Model file for the job. Use its own axes, mm. Coordinates: 2 decimals unless noted, no trailing zeros. Write each loop counter-clockwise with the first axis right and the second up, starting at its lowest first coordinate (ties: lowest second). Pieces come first, ordered by that corner, then holes. Notation, with made-up numbers: M 85.25,21.5 L 127.25,21.5 A3 cw 127.25,25.5 Z; hole C 25.25,17 d9. An arc over 180 degrees is marked long. One line per question, with ' | ' between items. Start each with the question number.
(1) Two-plate mould, pull along X, no slides. Class faces 1 (the face through (3.19, -39.37, 1.97)), 2 (the face through (103, 25, 4)), 3 (the face through (-28.24, 37.62, 1.97)): +X half, -X half, draft (parallel to the pull), parting line (faces both ways), or undercut.
(2) Wall check: probe 1 along Y at (x, z) = (56, 1.4); probe 2 along X at (y, z) = (4, 1.55); probe 3 along X at (y, z) = (-11, 0.2). Give the ranges that are in metal, low to high.
(3) Cut at A-A (z = 1.35). Write the cut outline in (x, y), plus the area to 3 significant figures.
(4) Cut at B-B (x = 131). Write the cut outline in (y, z).
(5) Cut at C-C (y = 32). Write the cut outline in (x, z).
(6) Flat gauge pins, fed straight in: pin 1 Ø1.2 at (y, z) = (4.5, 2) entering from +X; pin 2 Ø2 at (y, z) = (-7, 2.5) entering from -X. Where does each tip first touch, or does it go through?
Autodesk Inventor part; units mm, degrees
ref_plane "YZ Plane" through (0, 0, 0) normal (1, 0, 0) x (0, 1, 0)
ref_plane "XZ Plane" through (0, 0, 0) normal (0, 1, 0) x (-1, 0, 0)
ref_plane "XY Plane" through (0, 0, 0) normal (0, 0, 1) x (1, 0, 0)
sketch "Sketch1" plane through (0, 0, 0) normal (0, 0, 1) x (1, 0, 0)
  circle A0 centre (0, 0) radius 22.3333
  circle A1 centre (8.5222, 5.6951) radius 2
  circle A2 centre (0.671, -10.228) radius 2
  circle A3 centre (-9.1932, 4.5329) radius 2
  arc A4 (-33.8969, -20.2792) -> (36.2558, -15.6768) centre (0, 0) ccw
  arc A5 (39.2843, 4.1223) -> (-39.4862, -1.0454) centre (0, 0) ccw
  circle A6 centre (0, 0) radius 39.5
  line L0 (364.1325, 23.8889) -> (45.9013, 3.0114)
  line L1 (26.2679, 39.5) -> (334.9329, 39.5)
  line L2 (334.9329, 39.5) -> (334.9329, 0)
  line L3 (39.5, 10) -> (334.9329, 10)
  line L4 (334.9329, 10) -> (334.9329, 0)
  line L5 (334.9329, 39.5) -> (26.2679, 39.5)
  line L6 (0, 49.5) -> (334.9329, 49.5)
  line L7 (334.9329, 49.5) -> (334.9329, 39.5)
  arc A7 (39.1823, 5) -> (26.2679, 39.5) centre (0, 10) ccw
  arc A8 (0, 49.5) -> (-39.1823, 5) centre (0, 10) ccw
  line L8 (0, 0) -> (-39.5, 0)
  line L9 (-39.5, 0) -> (-39.5, 10)
  line L10 (39.5, 0) -> (39.5, 10)
  point P0 (0, 0)
  point P1 (-39.4862, -1.0454)
  point P2 (-33.8969, -20.2792)
  point P3 (36.2558, -15.6768)
extrude "Extrusion1" add sketch "Sketch1" along normal blind 4 contours A0 | A5 A6 A4 | L9 A8 A5 | A8 L6 L7 L1 A7 A5 | A7 L10 A6 A5 | A7 L1 L2 L0 L3 | L0 L2 L3
properties part number "lokiec"
Filled in:
1) face 1: parting line | face 2: draft | face 3: -X half
2) probe 1: 10 to 49.5 | probe 2: -39.5 to -11.12, -7.27 to 7.46, 9.58 to 39.5 | probe 3: -37.94 to -1.17, 2.52 to 37.94
3) outline: M -39.5,0 A39.5 ccw -39.49,-1.05 A39.5 ccw -33.9,-20.28 A39.5 ccw 36.26,-15.68 A39.5 ccw 39.5,0 L 39.5,10 L 334.93,10 L 334.93,49.5 L 0,49.5 A39.5 ccw -39.5,10 Z; hole C -9.19,4.53 d4; hole C 0.67,-10.23 d4; hole C 8.52,5.7 d4 | area: 17,700 mm²
4) outline: M 10,0 L 49.5,0 L 49.5,4 L 10,4 Z
5) outline: M -32.81,0 L 334.93,0 L 334.93,4 L -32.81,4 Z
6) pin 1: x = 39.5 | pin 2: x = -39.04
